Build history of the part. All positions in model axes, mm. Face numbers are marked on the shaded views. A direction names the side the tool comes from. Round coordinates to 2 decimals unless told otherwise and drop trailing zeros. Write each loop counter-clockwise with the first axis right and the second up, starting at its lowest first coordinate (ties: lowest second). Pieces come first, ordered by that corner, then holes. Notation, with made-up numbers: (84, -24) - (93, -24) arc R11 cw to (93, -7) - close; hole circle Ø9 at (50, 49). An arc over 180 degrees is marked (long way). One line per question, with ' | ' between items.
Autodesk Inventor part; units mm, degrees
ref_plane "YZ Plane" through (0, 0, 0) normal (1, 0, 0) x (0, 1, 0)
ref_plane "XZ Plane" through (0, 0, 0) normal (0, 1, 0) x (-1, 0, 0)
ref_plane "XY Plane" through (0, 0, 0) normal (0, 0, 1) x (1, 0, 0)
sketch "Skizze1" plane through (0, 0, 0) normal (0, 0, 1) x (1, 0, 0)
  line L0 (-16, 20) -> (16, 20)
  line L1 (16, 20) -> (16, -20)
  line L2 (16, -20) -> (-16, -20)
  line L3 (-16, -20) -> (-16, 20)
  line L4 (-16, 20) -> (16, -20) construction
  line L5 (16, 20) -> (-16, -20) construction
  point P0 (0, 0)
  dimension "d0" = 32
  dimension "d1" = 40
extrude "Extrusion1" add sketch "Skizze1" along normal blind 15
sketch "Skizze2" plane through (-16, -20, 0) normal (0, -1, 0) x (1, 0, 0)
  line L0 (0, 15) -> (32, 15)
  line L1 (0, 0) -> (0, 15)
  line L2 (32, 0) -> (0, 0)
  line L3 (32, 0) -> (32, 15)
  line L4 (32, 15) -> (0, 15)
  circle A0 centre (16, 15) radius 10
  point P0 (16, 0)
  dimension "d4" = 20
extrude "Extrusion2" cut sketch "Skizze2" against normal blind 15 contours A0 L0 | L0 A0
sketch "Skizze3" plane through (-16, -5, 0) normal (0, -1, 0) x (1, 0, 0)
  line L0 (0, 0) -> (0, 15)
  line L1 (32, 0) -> (0, 0)
  line L2 (32, 0) -> (32, 15)
  line L3 (26, 15) -> (32, 15)
  line L4 (0, 15) -> (6, 15)
  line L5 (6, 15) -> (26, 15)
  circle A0 centre (16, 15) radius 10.5
  point P0 (16, 0)
  dimension "d7" = 21
extrude "Extrusion3" cut sketch "Skizze3" against normal blind 5 contours A0 L3 L5 L4 | L4 L5 L3 A0
sketch "Skizze4" plane through (-16, 0, 0) normal (0, -1, 0) x (1, 0, 0)
  line L0 (5.5, 15) -> (26.5, 15)
  circle A0 centre (16, 15) radius 12.5
  point P0 (16, 0)
  dimension "d10" = 25
extrude "Extrusion4" cut sketch "Skizze4" against normal through all
sketch "Skizze5" plane through (0, 0, 15) normal (0, 0, 1) x (1, 0, 0)
  line L0 (-16, 20) -> (-16, -20)
  line L1 (-16, -20) -> (-10, -20)
  line L2 (-10, -20) -> (-10, -5)
  line L3 (10, -5) -> (10, -20)
  line L4 (10, -20) -> (16, -20)
  line L5 (16, -20) -> (16, 20)
  circle A0 centre (-13, -13) radius 1.8
  circle A1 centre (13, -13) radius 1.8
  point P0 (0, 0)
  dimension "d13" = 3.6
  dimension "d14" = 3.6
  dimension "d15" = 7
  dimension "d16" = 7
  dimension "d17" = 3
  dimension "d18" = 3
extrude "Extrusion5" cut sketch "Skizze5" against normal through all
sketch "Skizze6" plane through (0, 0, 0) normal (0, 0, -1) x (-1, 0, 0)
  line L0 (12.5, 20) -> (16, 20)
  line L1 (16, 20) -> (16, 11.5)
  line L2 (16, 20) -> (16, -20)
  line L3 (16, 11.5) -> (-16, 11.5)
  line L4 (-16, -20) -> (-16, 20)
  line L5 (-16, 20) -> (16, 20)
  point P0 (0, 0)
  dimension "d21" = 8.5
extrude "Extrusion6" cut sketch "Skizze6" against normal blind 22.5
properties part number "oberteil (1)"
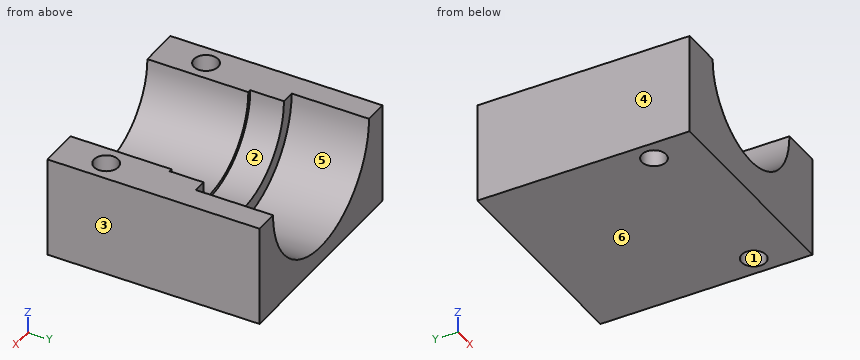
Q1. Which spindle directions (+Z, -Z, +X, -X, +Y, -Y) get a long thin tool onto all of the face, cutting with end or side? Do the marked faces 1 and 2. Say none if no direction does.
Found:
face 1: +Z, -Z | face 2: +Z, +Y
Q2. Saw through at D-D, the plane z = 1.75. List the corners of the cut face in (x, y).
Found:
outline: (-16, -20) - (16, -20) - (16, 11.5) - (-16, 11.5) - close; hole circle Ø3.6 at (-13, -13); hole circle Ø3.6 at (13, -13)
Q3. Saw through at A-A, the plane y = -13. List the corners of the cut face in (x, z), then the cut area to 3 significant figures.
Found:
outline: (-16, 0) - (-14.8, 0) - (-14.8, 15) - (-16, 15) - close; (-11.2, 0) - (11.2, 0) - (11.2, 15) - (10, 15) arc R10 cw to (-10, 15) - (-11.2, 15) - close; (14.8, 0) - (16, 0) - (16, 15) - (14.8, 15) - close | area: 215 mm^2
Q4. Drill centre lines: L1, parallel to Y at x = -13, z = 8; L2, parallel to X at y = -11.5, z = 7; L3, parallel to Y at x = 7.5, z = 7. Where is each one in solid material? Low to high. Write a range as from..to.
Found:
L1: -20..-14.8, -11.2..11.5 | L2: -16..-13.99, -12.01..-6, 6..12.01, 13.99..16 | L3: -20..0
Q5. Drop flat-ended pins along their axis: pin 1 (6 mm diameter, centred on x = -3.5, y = -14.5, fed in from +Z); pin 2 (1 mm diameter, centred on x = 7.5, y = 6.5, fed in from +Z). Give the stop position or say it passes through.
Found:
pin 1: z = 7.4 | pin 2: z = 5.4
Q6. Saw through at B-B, the plane z = 7.5. List the corners of the cut face in (x, y), then the cut area to 3 significant figures.
Found:
outline: (-16, -20) - (-6.61, -20) - (-6.61, -5) - (-7.35, -5) - (-7.35, 0) - (-10, 0) - (-10, 11.5) - (-16, 11.5) - close; (6.61, -20) - (16, -20) - (16, 11.5) - (10, 11.5) - (10, 0) - (7.35, 0) - (7.35, -5) - (6.61, -5) - close; hole circle Ø3.6 at (-13, -13); hole circle Ø3.6 at (13, -13) | area: 486 mm^2
Q7. Pull direction X, two halves, no side cores. Call the marked faces 3, 4, 5 and 6: +X half, -X half, draft (parallel to the pull), parting line (faces both ways), or undercut.
Found:
face 3: +X half | face 4: -X half | face 5: undercut | face 6: draft
Q8. Saw through at C-C, the plane x = 13. List the corners of the cut face in (y, z).
Found:
outline: (-20, 0) - (-14.8, 0) - (-14.8, 15) - (-20, 15) - close; (-11.2, 0) - (11.5, 0) - (11.5, 15) - (-11.2, 15) - close
